Here's how the part is built. I have some questions about the finished solid (model axes, mm). A direction names the side the tool comes from. Coordinates: 2 decimals unless noted, no trailing zeros. Order: outer loops, then holes, each group sorted by start corner. A loop starts at its lowest first (then second) coordinate and runs counter-clockwise, first axis right, second up. Notation, with made-up numbers: M -19.5,-35 L 8.5,-35 A29 ccw 8.5,-7 Z; hole C -34,37 d5. An arc over 180 degrees is marked long. Answer as CSV lines item,"result". Start each with the question number.
```python
from build123d import *

# Parameters (mm, degrees)
F0_R      = 2
F1_DEPTH  = 40.5
F2_W      = 47.270983
F2_H      = 47.419636
F3_DEPTH  = 3
F4_W      = 47.122335
F4_H      = 3.418969
F5_DEPTH  = 50
F6_W      = 2
F6_H      = 44
F7_DEPTH  = 20
F8_W      = 2
F8_H      = 44
F9_DEPTH  = 20
F10_W     = 42
F10_H     = 18
F11_DEPTH = 25
F12_W     = 42
F12_H     = 18
F13_DEPTH = 25


with BuildPart() as f1:
    # F0 (on Top) → F1 (new body)
    with BuildSketch(Plane.XY):
        with Locations((-19.125001, -21.954547)):
            Circle(F0_R)
        with Locations((20.874999, 18.045453)):
            Circle(F0_R)
        with Locations((20.874999, -21.954547)):
            Circle(F0_R)
        with Locations((-19.125001, 18.045453)):
            Circle(F0_R)
    extrude(amount=F1_DEPTH)

    # F2 (on Top) → F3 (join)
    with BuildSketch(Plane.XY):
        with Locations((0.872621, -1.915443)):
            Rectangle(F2_W, F2_H)
    extrude(amount=-F3_DEPTH)

    # F4 (on Top) → F5 (join)
    with BuildSketch(Plane.XY):
        with Locations((0.946948, -24.064426)):
            Rectangle(F4_W, F4_H)
    extrude(amount=-F5_DEPTH)

    # F6 (on face) → F7 (join)
    with BuildSketch(Plane(origin=(0, 0, -3), x_dir=(1, 0, 0), z_dir=(0, 0, -1))):
        with Locations((23.508113, 0.205625)):
            Rectangle(F6_W, F6_H)
    extrude(amount=F7_DEPTH)

    # F8 (on face) → F9 (join)
    with BuildSketch(Plane(origin=(0, 0, -3), x_dir=(1, 0, 0), z_dir=(0, 0, -1))):
        with Locations((-21.76287, 0.205625)):
            Rectangle(F8_W, F8_H)
    extrude(amount=F9_DEPTH)

    # F10 (on face) → F11 (cut)
    with BuildSketch(Plane.YZ.offset(24.508113)):
        with Locations((-1.205625, -12)):
            Rectangle(F10_W, F10_H)
    extrude(amount=-F11_DEPTH, mode=Mode.SUBTRACT)

    # F12 (on face) → F13 (cut)
    with BuildSketch(Plane(origin=(-22.76287, 0, 0), x_dir=(0, -1, 0), z_dir=(-1, 0, 0))):
        with Locations((1.205625, -12)):
            Rectangle(F12_W, F12_H)
    extrude(amount=-F13_DEPTH, mode=Mode.SUBTRACT)


solid = f1.part
```
1) Will these pins go through, and if not, where does the flat tip stop? pin 1 Ø23.5 at (x, y) = (10, 3) entering from +Z; pin 2 Ø2 at (x, y) = (23.5, -9) entering from -Z; pin 3 Ø16 at (y, z) = (-3, -12.5) entering from +X; pin 4 Ø6 at (x, y) = (7, -17) entering from -Z.
2) Which directions (+Z, -Z, +X, -X, +Y, -Y) give clear straight access to the entire face, cutting with the end or side of a thin tool? Please do faces 5 (the face through (-20.763, 6, -22)), 6 (the face through (21, 18, 40.5)), 7 (the face through (24, -1, -21)), 8 (the face through (22, -20.3, 20)), 9 (the face through (1, -24, -50)).
3) Suppose I cut it at A-A on z = -13. Please give me the cut outline in (x, y).
4) Suppose I cut it at C-C on x = -11. Please give me the cut outline in (y, z), plus the area to 3 significant figures.
5) I need wall thicknesses on line 1 (X direction, y = -19.5, z = -22); line 2 (Z direction, x = -8.5, y = 15.5); line 3 (Y direction, x = -20, z = -7). Which ranges of each line are inside material? Lowest first, please. Write a range as [from, to].
6) If we mould it in two halves opening along Y, with no side actions, what happens to faces 1 (the face through (-22, -1, -21)), 2 (the face through (-1, 21.794, -2)), 3 (the face through (1, -25.774, -25)), 4 (the face through (-22.614, -24, -30))? For each: released by +Y, released by -Y, zero draft, split by the parting line, or undercut.
7) Suppose I cut it at D-D on z = 12.5. Please give me the cut outline in (x, y) (3 decimals), plus the area to 3 significant figures.
8) Suppose I cut it at B-B on y = 14.5. Please give me the cut outline in (x, z).
Output:
1,pin 1,"z = 0"
1,pin 2,"z = -23"
1,pin 3,"through"
1,pin 4,"z = -3"
2,face 5,"-Z, +Y"
2,face 6,"+Z, +X, -X, +Y, -Y"
2,face 7,"+X, -X"
2,face 8,"+Z"
2,face 9,"-Z, +X, -X, +Y, -Y"
3,outline,"M -22.76,19.79 L -20.76,19.79 L -20.76,21.79 L -22.76,21.79 Z; M -22.61,-25.77 L 24.51,-25.77 L 24.51,-22.35 L -22.61,-22.35 Z; M 22.51,19.79 L 24.51,19.79 L 24.51,21.79 L 22.51,21.79 Z"
4,outline,"M -25.77,-50 L -22.35,-50 L -22.35,-3 L 21.79,-3 L 21.79,0 L -25.77,0 Z"
4,area,"303 mm²"
5,line 1,"[-22.76, -20.76], [22.51, 24.51]"
5,line 2,"[-3, 0]"
5,line 3,"[-25.77, -22.35]"
6,face 1,"undercut"
6,face 2,"released by +Y"
6,face 3,"released by -Y"
6,face 4,"zero draft"
7,outline,"C -19.125,-21.955 d4; C -19.125,18.045 d4; C 20.875,-21.955 d4; C 20.875,18.045 d4"
7,area,"50.3 mm²"
8,outline,"M -22.76,-23 L -20.76,-23 L -20.76,-21 L -22.76,-21 Z; M -22.76,-3 L 24.51,-3 L 24.51,0 L -22.76,0 Z; M 22.51,-23 L 24.51,-23 L 24.51,-21 L 22.51,-21 Z"
